The listing builds one solid part. Answer for the finished solid, in the listing's coordinates (mm). Face numbers are marked on the shaded views. A direction names the side the tool comes from. Give positions to 0.01 mm unless a question says otherwise; leave off trailing zeros. Loops run counter-clockwise (first coordinate to the right, second up) from the corner with the lowest first, then second, coordinate; pieces in that order, holes last.
Item 1: Section D-D, the plane y = 34 is taken. Give the vertices of the cut face in (x, z).
Item 2: A tool of negligible diameter and unlimited length cuts with its end or side. For the marked faces 1 and 2, from which of +Z, -Z, +X, -X, +Y, -Y can it reach the whole face along a straight path? Write none if from no direction.
Item 3: Consider line 1 along Z through (x, y) = (4.4, 25.4) (3 decimals); line 2 along Y through (x, z) = (23, 34). Determine where each line is inside the solid, lowest interval first.
Item 4: Each of these flat-tipped pins is pushed along its axis until it touches: pin 1 Ø6 at (x, z) = (7, 28.5) entering from -Y; pin 2 Ø10 at (x, z) = (33, 24) entering from +Y; pin 3 Ø10 at (y, z) = (29.5, 16) entering from +X. Where does it stop, or does it pass through?
Item 5: Section A-A, the plane y = 25.4 is taken. Give the vertices of the cut face in (x, z) (3 decimals), and give its area (3 significant figures).
Item 6: The mould has two halves that part along X. Classify the marked faces 3, 4 and 5: pulls with the +X half, pulls with the -X half, needs draft (parallel to the pull), parting line crosses it, or undercut.
Item 7: Section C-C, the plane z = 24.5 is taken. Give the vertices of the cut face in (x, y).
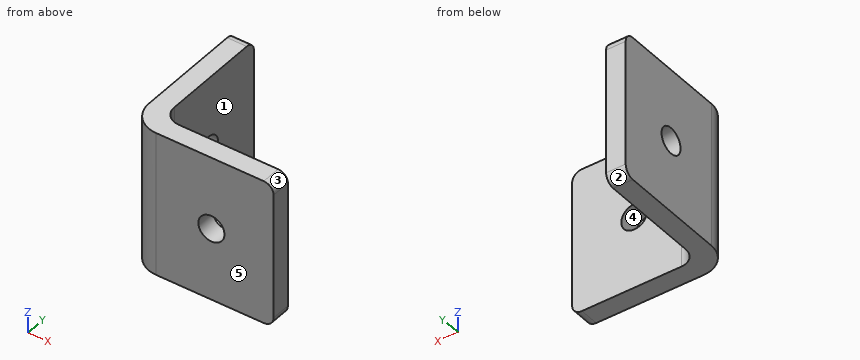
from build123d import *

# Parameters (mm, degrees)
F1_DEPTH = 44.45
F2_R     = 4
F3_DEPTH = 6
F4_R     = 4
F5_DEPTH = 6
F6_R     = 3


with BuildPart() as f1:
    # F0 (on Top) → F1 (new body)
    with BuildSketch(Plane.XY):
        with BuildLine():
            Line((6, 44.45), (0, 44.45))
            Line((0, 44.45), (0, 8.5))
            ThreePointArc((0, 8.5), (2.489592, 2.489592), (8.5, 0))
            Line((8.5, 0), (44.45, 0))
            Line((44.45, 0), (44.45, 6))
            Line((44.45, 6), (11, 6))
            ThreePointArc((11, 6), (7.464466, 7.464466), (6, 11))
            Line((6, 11), (6, 44.45))
        make_face()
    extrude(amount=F1_DEPTH)

    # F2 (on face) → F3 (cut, through all)
    with BuildSketch(Plane.YZ.offset(6)):
        with Locations((25.4, 22.225)):
            Circle(F2_R)
    extrude(amount=-F3_DEPTH, mode=Mode.SUBTRACT)

    # F4 (on face) → F5 (cut, through all)
    with BuildSketch(Plane.XZ):
        with Locations((25.4, 22.225)):
            Circle(F4_R)
    extrude(amount=-F5_DEPTH, mode=Mode.SUBTRACT)

    # F6
    f6_edges = [f1.edges().sort_by_distance(p)[0] for p in [
        (44.45, 3, 44.45),
        (44.45, 3, 0),
        (3, 44.45, 0),
        (3, 44.45, 44.45),
    ]]
    fillet(f6_edges, radius=F6_R)


solid = f1.part
Worked answers:
1. outline: (0, 0) - (6, 0) - (6, 44.45) - (0, 44.45) - close
2. face 1: +Z, -Z, +X, +Y
2. face 2: -Z, +X, -X, +Y
3. line 1: z = 0 to 18.225, 26.225 to 44.45
3. line 2: y = 0 to 6
4. pin 1: stops at y = 0
4. pin 2: stops at y = 6
4. pin 3: stops at x = 6
5. outline: (0, 0) - (6, 0) - (6, 18.225) - (0, 18.225) - close; (0, 26.225) - (6, 26.225) - (6, 44.45) - (0, 44.45) - close
5. area: 219 mm2
6. face 3: pulls with the +X half
6. face 4: undercut
6. face 5: needs draft
7. outline: (0, 8.5) arc R8.5 ccw to (8.5, 0) - (22.11, 0) - (22.11, 6) - (11, 6) arc R5 cw to (6, 11) - (6, 22.11) - (0, 22.11) - close; (0, 28.69) - (6, 28.69) - (6, 44.45) - (0, 44.45) - close; (28.69, 0) - (44.45, 0) - (44.45, 6) - (28.69, 6) - close
